from build123d import *

# Parameters (mm, degrees)
CROQUIS1_R              = 1.53
CROQUIS1_R_2            = 1.837919526
CROQUIS1_R_3            = 1.597275243
CROQUIS1_R_4            = 1.5
SALIENTE_EXTRUIR1_DEPTH = 3
CROQUIS2_R              = 1.8
CORTAR_EXTRUIR1_DEPTH   = 10


with BuildPart() as part:
    # Croquis1 → Saliente-Extruir1 (new body)
    with BuildSketch(Plane(origin=(0, 0, 0), x_dir=(1, 0, 0), z_dir=(0, 1, 0))):
        Polygon((-26.514888395, -10.582637626), (-26.514888395, -7.527182045), (-40.886979894, -7.527182045), (-58.77250276, -7.527182045), (-58.77250276, 15.200062733), (-41.405808266, 15.200062733), (-25.724953766, 15.200062733), (-14.794888395, 24.417362374), (0.205111605, 24.417362374), (11.925111605, 14.417362374), (11.925111605, -10.582637626), (0.205111605, -20.582637626), (-14.794888395, -20.582637626), align=None)
        with Locations((-11.884888395, -14.457637626)):
            Circle(CROQUIS1_R, mode=Mode.SUBTRACT)
        with Locations((-2.704888395, -14.457637626)):
            Circle(CROQUIS1_R, mode=Mode.SUBTRACT)
        with Locations((5.705111605, 3.842362374)):
            Circle(CROQUIS1_R_2, mode=Mode.SUBTRACT)
        with Locations((-43.610544187, 3.842362374)):
            Circle(CROQUIS1_R_3, mode=Mode.SUBTRACT)
        with Locations((-6.044888395, 3.842362374)):
            Circle(CROQUIS1_R_4, mode=Mode.SUBTRACT)
        with Locations((-6.044888395, 10.008584025)):
            Circle(CROQUIS1_R_4, mode=Mode.SUBTRACT)
        with Locations((-6.044888395, -2.323859276)):
            Circle(CROQUIS1_R_4, mode=Mode.SUBTRACT)
        with Locations((-56.194888395, 10.008584025)):
            Circle(CROQUIS1_R_4, mode=Mode.SUBTRACT)
        with Locations((-56.194888395, -2.323859276)):
            Circle(CROQUIS1_R_4, mode=Mode.SUBTRACT)
        with BuildLine():
            Line((-40.195554385, 11.342362374), (-20.294888395, 11.342362374))
            ThreePointArc((-20.294888395, 11.342362374), (-12.794888395, 3.842362374), (-20.294888395, -3.657637626))
            Line((-20.294888395, -3.657637626), (-40.195554385, -3.657637626))
            Line((-40.195554385, -3.657637626), (-40.195554385, 11.342362374))
        make_face(mode=Mode.SUBTRACT)
    extrude(amount=SALIENTE_EXTRUIR1_DEPTH)

    # Croquis2 → Cortar-Extruir1 (cut)
    with BuildSketch(Plane(origin=(0, 3, 0), x_dir=(1, 0, 0), z_dir=(0, 1, 0))):
        with Locations((-11.039224955, 20.862391136)):
            Circle(CROQUIS2_R)
        with Locations((-1.039224955, 20.862391136)):
            Circle(CROQUIS2_R)
    extrude(amount=-CORTAR_EXTRUIR1_DEPTH, mode=Mode.SUBTRACT)


solid = part.part
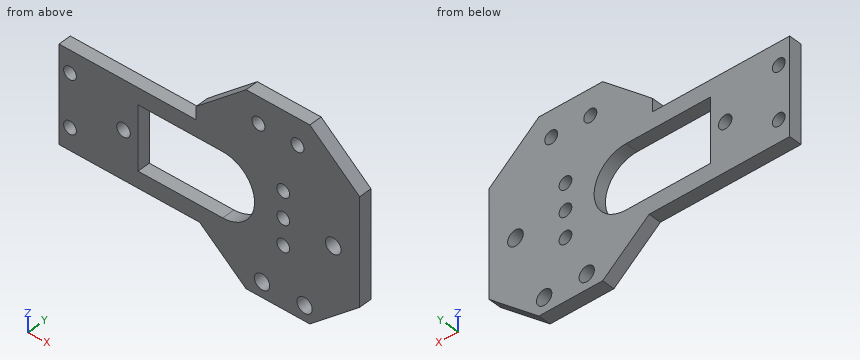
The model under review builds one solid part; all positions refer to its coordinate system, in mm. Give positions to 0.01 mm unless a question says otherwise; leave off trailing zeros. Loops run counter-clockwise (first coordinate to the right, second up) from the corner with the lowest first, then second, coordinate; pieces in that order, holes last. Notation, with made-up numbers: (87, 29.5) -> (97, 29.5) arc R11 cw to (97, 39.5) -> close; hole circle Ø2 at (49.25, 72). An arc over 180 degrees is marked (long way). Answer as a JSON object with one key per item and string values. Group by question number.
Q1. Wall thickness on line 1 along Z through (x, y) = (-37, 0.7); line 2 along X through (y, z) = (1.05, -20); line 3 along Z through (x, y) = (-55, 1.6): over which ranges is each line inside the solid? List them lowest first.
Q2. Take a section at B-B (y = 1.8). State how many separate pieces and enclosed holes the cut face has, plus the area to 3 significant figures.
Q3. Take a section at D-D (x = -18). Write out the cut boundary in (y, z), plus the area to 3 significant figures.
Q4. Take a section at A-A (x = -38). Write out the cut boundary in (y, z), plus the area to 3 significant figures.
Q5. Take a section at C-C (z = -20). Write out the cut boundary in (x, y), plus the area to 3 significant figures.
Q6. Insertion check: pin 1 (5 mm diameter, centred on x = -11.88, z = 14.46, fed in from +Y); pin 2 (0.9 mm diameter, centred on x = -37.5, y = 1.5, fed in from +Z); pin 3 (2.5 mm diameter, centred on x = -56.19, z = -10.01, fed in from -Y); pin 4 (0.9 mm diameter, centred on y = 1, z = 10, fed in from -X). Each pin has a flat end and moves straight along its axis. Give the tip position at first contact, or say it passes through.
Answer below:
{
 "1": {"line 1": "z = -15.2 to -11.34, 3.66 to 7.53", "line 2": "x = -20.03 to -12.62, -9.46 to -2.62, 0.54 to 5.38", "line 3": "z = -15.2 to -10.92, -9.1 to 1.42, 3.23 to 7.53"},
 "2": {"separate pieces": "1", "enclosed holes": "12", "area": "1,750 mm2"},
 "3": {"outline": "(0, -21.71) -> (3, -21.71) -> (3, -10.98) -> (0, -10.98) -> close; (0, 3.3) -> (3, 3.3) -> (3, 17.85) -> (0, 17.85) -> close", "area": "75.8 mm2"},
 "4": {"outline": "(0, -15.2) -> (3, -15.2) -> (3, -11.34) -> (0, -11.34) -> close; (0, 3.66) -> (3, 3.66) -> (3, 7.53) -> (0, 7.53) -> close", "area": "23.2 mm2"},
 "5": {"outline": "(-20.03, 0) -> (-12.62, 0) -> (-12.62, 3) -> (-20.03, 3) -> close; (-9.46, 0) -> (-2.62, 0) -> (-2.62, 3) -> (-9.46, 3) -> close; (0.54, 0) -> (5.38, 0) -> (5.38, 3) -> (0.54, 3) -> close", "area": "57.3 mm2"},
 "6": {"pin 1": "stops at y = 3", "pin 2": "stops at z = 7.53", "pin 3": "passes through", "pin 4": "stops at x = -26.51"}
}
